from build123d import *

# Parameters (mm, degrees)
SKETCH1_W           = 200
SKETCH1_H           = 110
BOSS_EXTRUDE1_DEPTH = 3
SKETCH2_W           = 200
SKETCH2_H           = 110
SKETCH2_W_2         = 194
SKETCH2_H_2         = 104
BOSS_EXTRUDE2_DEPTH = 12
SKETCH3_R           = 1.4
CUT_EXTRUDE2_DEPTH  = 3
SKETCH5_R           = 7
CUT_EXTRUDE3_DEPTH  = 3


with BuildPart() as part:
    # Sketch1 → Boss-Extrude1 (new body)
    with BuildSketch(Plane.XY):
        with Locations((3.991596639, -23.697478992)):
            Rectangle(SKETCH1_W, SKETCH1_H)
    extrude(amount=BOSS_EXTRUDE1_DEPTH)

    # Sketch2 → Boss-Extrude2 (add)
    with BuildSketch(Plane.XY.offset(3)):
        with Locations((3.991596639, -23.697478992)):
            Rectangle(SKETCH2_W, SKETCH2_H)
        with Locations((3.991596639, -23.697478992)):
            Rectangle(SKETCH2_W_2, SKETCH2_H_2, mode=Mode.SUBTRACT)
    extrude(amount=BOSS_EXTRUDE2_DEPTH)

    # Sketch3 → Cut-Extrude2 (cut)
    with BuildSketch(Plane.XY.offset(3)):
        with Locations((-89.008403361, 24.302521008)):
            Circle(SKETCH3_R)
        with Locations((-89.008403361, -71.697478992)):
            Circle(SKETCH3_R)
        with Locations((96.991596639, 24.302521008)):
            Circle(SKETCH3_R)
        with Locations((96.991596639, -71.697478992)):
            Circle(SKETCH3_R)
    extrude(amount=-CUT_EXTRUDE2_DEPTH, mode=Mode.SUBTRACT)

    # Sketch5 → Cut-Extrude3 (cut)
    with BuildSketch(Plane.XY.offset(3)):
        with Locations((-51.008403361, -1.697478992)):
            Circle(SKETCH5_R)
    extrude(amount=-CUT_EXTRUDE3_DEPTH, mode=Mode.SUBTRACT)


solid = part.part
Here's how the part is built. I have some questions about the finished solid (model axes, mm). A direction names the side the tool comes from. Round coordinates to 2 decimals unless told otherwise and drop trailing zeros. Order: outer loops, then holes, each group sorted by start corner. A loop starts at its lowest first (then second) coordinate and runs counter-clockwise, first axis right, second up. Notation, with made-up numbers: M 59.25,-9.75 L 118.25,-9.75 A10 cw 118.25,4.25 Z; hole C 76.25,-11.5 d10. An arc over 180 degrees is marked long. One line per question, with ' | ' between items.
1) I'm going to push flat-ended pins straight in: pin 1 Ø3.5 at (x, y) = (96.99, -71.7) entering from +Z; pin 2 Ø2 at (x, y) = (-89.01, -71.7) entering from -Z. Where does each tip first touch, or does it pass through?
Checked values:
pin 1: stops at z = 3 | pin 2: passes through
2) We'd pull the mould along X, two halves only. Please class faces 3 (the flat face through (3, -23, 3)), 4 (the flat face through (103.992, -24, 7)), 5 (the flat face through (3, 31.303, 7)), 6 (the flat face through (-96.008, -24, 7)): released by +X, released by -X, zero draft, split by the parting line, or undercut.
Checked values:
face 3: undercut | face 4: released by +X | face 5: zero draft | face 6: released by -X
3) Imagine slicing it at C-C, the plane y = -18.5. Write out the boundary of the cut face in (x, z), plus the area to 3 significant figures.
Checked values:
outline: M -96.01,0 L 103.99,0 L 103.99,15 L 100.99,15 L 100.99,3 L -93.01,3 L -93.01,15 L -96.01,15 Z | area: 672 mm²
4) Imagine slicing it at A-A, the plane z = 8. Write out the boundary of the cut face in (x, y), plus the area to 3 significant figures.
Checked values:
outline: M -96.01,-78.7 L 103.99,-78.7 L 103.99,31.3 L -96.01,31.3 Z; hole M -93.01,-75.7 L 100.99,-75.7 L 100.99,28.3 L -93.01,28.3 Z | area: 1,820 mm²
5) Imagine slicing it at B-B, the plane x = -49. Write out the boundary of the cut face in (y, z), plus the area to 3 significant figures.
Checked values:
outline: M -78.7,0 L -8.4,0 L -8.4,3 L -75.7,3 L -75.7,15 L -78.7,15 Z; M 5.01,0 L 31.3,0 L 31.3,15 L 28.3,15 L 28.3,3 L 5.01,3 Z | area: 362 mm²
6) I need wall thicknesses on line 1 (X direction, y = -39, z = 8.5); line 2 (Y direction, x = 16.5, z = 13.25); line 3 (Z direction, x = -18.5, y = 8.5). Which ranges of each line are inside material? Lowest first, please.
Checked values:
line 1: x = -96.01 to -93.01, 100.99 to 103.99 | line 2: y = -78.7 to -75.7, 28.3 to 31.3 | line 3: z = 0 to 3
7) On a 3-axis mill with a long thin cutter (end or side, diameter ignored), from which of +Z, -Z, +X, -X, +Y, -Y can I reach the whole of each face in a straight line? I mean faces 1 (the flat face through (3, -75.697, 9)), 2 (the cylindrical face through (-47.78, -7.91, 1.52)). Say none if no direction works.
Checked values:
face 1: +Z | face 2: +Z, -Z
